Source: CAD feature listing. Evaluate the final solid. Frame: model axes, mm. Face numbers are marked on the shaded views. A direction names the side the tool comes from. Give positions to 0.01 mm unless a question says otherwise; leave off trailing zeros. Write each loop counter-clockwise with the first axis right and the second up, starting at its lowest first coordinate (ties: lowest second). Pieces come first, ordered by that corner, then holes. Notation, with made-up numbers: (0.25, 11.5) -> (24.25, 11.5) arc R15 ccw to (24.25, 38.5) -> close; hole circle Ø3 at (-37, 64). An arc over 180 degrees is marked (long way). Use one line per item in the form item = value. Start each with the question number.
(1) Cut plane C-C, the plane x = -34.5. Output: boundary loops of the cut face in (y, z), and give its area (3 significant figures).
(2) Material intervals for line 1 along Y through (x, z) = (-6.5, 136); line 2 along X through (y, z) = (26, 52.5); line 3 along Z through (x, y) = (-4, 20.5), sorted ascending. Write a range as from..to.
(3) Draft query along X for the marked faces 3, 4, 5 and 6. Return one class per face: pulls with the +X half, pulls with the -X half, needs draft (parallel to the pull), parting line crosses it, or undercut.
(4) Cut plane A-A, the plane y = 42.5. Output: boundary loops of the cut face in (x, z), and give its area (3 significant figures).
(5) Set-up query: the marked faces 1 and 2. Return all of +Z, -Z, +X, -X, +Y, -Y with unobstructed straight access to the full face (end or side cutting, diameter ignored); none if empty.
(6) Cut plane B-B, the plane z = 79.5. Output: boundary loops of the cut face in (x, y).
from build123d import *

# Parameters (mm, degrees)
F0_W     = 50.8
F0_H     = 50.8
F0_W_2   = 41.275
F0_H_2   = 41.275
F1_DEPTH = 381
F3_DEPTH = 50.801


with BuildPart() as f1:
    # F0 (on Top) → F1 (new body)
    with BuildSketch(Plane.XY):
        with Locations((-25.4, 25.4)):
            Rectangle(F0_W, F0_H)
        with Locations((-25.4, 25.4)):
            Rectangle(F0_W_2, F0_H_2, mode=Mode.SUBTRACT)
    extrude(amount=F1_DEPTH)

    # F2 (on face) → F3 (cut, through all)
    with BuildSketch(Plane.XZ):
        Polygon((0, 372.042589), (0, 381), (-50.8, 381), align=None)
    extrude(amount=-F3_DEPTH, mode=Mode.SUBTRACT)


solid = f1.part
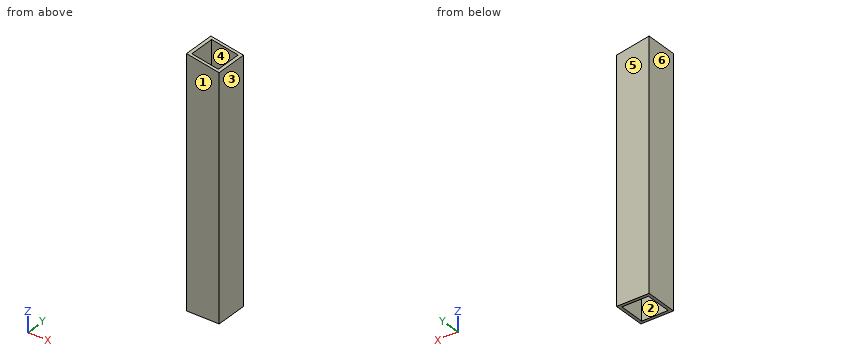
Geometry says:
q1.outline = (0, 0) -> (4.76, 0) -> (4.76, 378.13) -> (0, 378.13) -> close; (46.04, 0) -> (50.8, 0) -> (50.8, 378.13) -> (46.04, 378.13) -> close
q1.area = 3,600 mm^2
q2.line_1 = 0..4.76, 46.04..50.8
q2.line_2 = -50.8..-46.04, -4.76..0
q2.line_3 = 0..372.75
q3.face_3 = pulls with the +X half
q3.face_4 = undercut
q3.face_5 = needs draft
q3.face_6 = pulls with the -X half
q4.outline = (-50.8, 0) -> (-46.04, 0) -> (-46.04, 380.16) -> (-50.8, 381) -> close; (-4.76, 0) -> (0, 0) -> (0, 372.04) -> (-4.76, 372.88) -> close
q4.area = 3,590 mm^2
q5.face_1 = +Z, -Z, +X, -X, -Y
q5.face_2 = +Z, -Z
q6.outline = (-50.8, 0) -> (0, 0) -> (0, 50.8) -> (-50.8, 50.8) -> close; hole (-46.04, 4.76) -> (-4.76, 4.76) -> (-4.76, 46.04) -> (-46.04, 46.04) -> close
